```python
from build123d import *

# Parameters (mm, degrees)
SKETCH3_R           = 19.05
SKETCH3_R_2         = 2.159
BOSS_EXTRUDE1_DEPTH = 1.27


with BuildPart() as part:
    # Sketch2 → Revolve1 (revolve)
    with BuildSketch(Plane.XY, mode=Mode.PRIVATE) as revolve1_sk:
        Polygon((3.302, 35.814), (4.953, 35.814), (4.953, 28.702), (19.05, 28.702), (19.05, 18.669), (19.05, 17.399), (19.05, 7.366), (3.302, 7.366), align=None)
    revolve(revolve1_sk.sketch.rotate(Axis((0, 35.814, 0), (0, -1, 0)), 180), axis=Axis((0, 35.814, 0), (0, -1, 0)))

    # Sketch3 → Boss-Extrude1 (add)
    with BuildSketch(Plane(origin=(0, 17.399, 0), x_dir=(1, 0, 0), z_dir=(0, 1, 0))):
        with BuildLine():
            Line((-17.526, 22.225), (17.526, 22.225))
            ThreePointArc((17.526, 22.225), (20.848694765, 20.848694765), (22.225, 17.526))
            Line((22.225, 17.526), (22.225, -17.526))
            ThreePointArc((22.225, -17.526), (20.848694765, -20.848694765), (17.526, -22.225))
            Line((17.526, -22.225), (-17.526, -22.225))
            ThreePointArc((-17.526, -22.225), (-20.848694765, -20.848694765), (-22.225, -17.526))
            Line((-22.225, -17.526), (-22.225, 17.526))
            ThreePointArc((-22.225, 17.526), (-20.848694765, 20.848694765), (-17.526, 22.225))
        make_face()
        with Locations(Location((0, 0, 0), (0, 0, 180))):
            Circle(SKETCH3_R, mode=Mode.SUBTRACT)
        with Locations(Location((-17.526, -17.526, 0), (0, 0, 270))):
            Circle(SKETCH3_R_2, mode=Mode.SUBTRACT)
        with Locations(Location((17.526, -17.526, 0), (0, 0, 270))):
            Circle(SKETCH3_R_2, mode=Mode.SUBTRACT)
        with Locations(Location((-17.526, 17.526, 0), (0, 0, 270))):
            Circle(SKETCH3_R_2, mode=Mode.SUBTRACT)
        with Locations(Location((17.526, 17.526, 0), (0, 0, 270))):
            Circle(SKETCH3_R_2, mode=Mode.SUBTRACT)
    extrude(amount=BOSS_EXTRUDE1_DEPTH)


solid = part.part
```
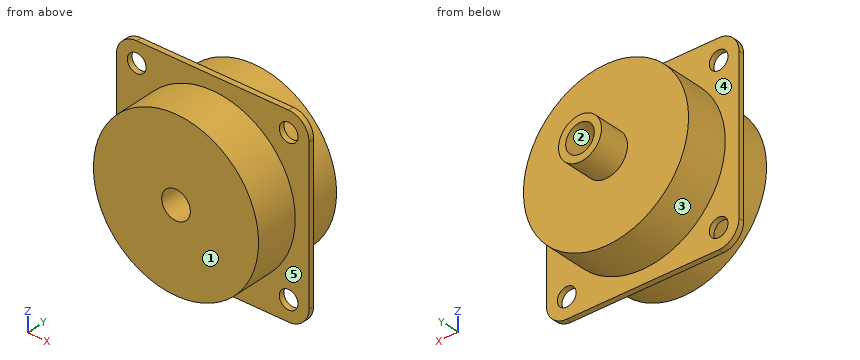
For this review, take the finished solid that the model builds, in its own axes (mm). Face numbers are marked on the shaded views. A direction names the side the tool comes from. Give positions to 0.01 mm unless a question says otherwise; leave off trailing zeros. Loops run counter-clockwise (first coordinate to the right, second up) from the corner with the lowest first, then second, coordinate; pieces in that order, holes last. Notation, with made-up numbers: M -26,-39 L 26,-39 A23 ccw 26,-22 Z; hole C 60.5,26 d8. An arc over 180 degrees is marked long. One line per item, written item: value. Start each with the question number.
Q1. Machinability: for the marked faces 4 and 5, which of the approach directions +Z, -Z, +X, -X, +Y, -Y give a long, thin tool a straight path to every point of the face, cutting with its end or side? Answer none if there is none.
Q2. Add section D-D (z = -9). Give the boundary of the cut face in (x, y) (3 decimals).
Q3. Add section B-B (z = 0). Give the boundary of the cut face in (x, y) (3 decimals), and give its area (3 significant figures).
Q4. Draft analysis for pull direction Z (two halves, no side actions). For the marked faces 1, 2 and 3, state which applies: released by +Z, released by -Z, zero draft, split by the parting line, or undercut.
Q5. Add section A-A (x = 0). Give the boundary of the cut face in (y, z) (3 decimals), and give its area (3 significant figures).
Q6. Clearance check with flat-ended pins moving along their axes: pin 1 Ø4 at (y, z) = (29, -6) entering from +X; pin 2 Ø5.5 at (x, z) = (17.526, 17.526) entering from -Y; pin 3 Ø8 at (y, z) = (30.5, -4.5) entering from -X; pin 4 Ø3.5 at (x, z) = (-17.526, 17.526) entering from +Y. State where each tip first meets the part, or that it passes through.
Q7. Add section C-C (y = 23). Give the boundary of the cut face in (x, z).
Q8. For L1, parallel to Y at x = -15, z = -20; L2, parallel to Y at x = 5, z = 8.5; L3, parallel to Z at x = 18, y = 18, list the stretches that pass through material, from the lowest coordinate up.
Reply:
1. face 4: +Y
1. face 5: -Y
2. outline: M -22.225,17.399 L -16.79,17.399 L -16.79,7.366 L 16.79,7.366 L 16.79,17.399 L 22.225,17.399 L 22.225,18.669 L 16.79,18.669 L 16.79,28.702 L -16.79,28.702 L -16.79,18.669 L -22.225,18.669 Z
3. outline: M -22.225,17.399 L -19.05,17.399 L -19.05,7.366 L -3.302,7.366 L -3.302,35.814 L -4.953,35.814 L -4.953,28.702 L -19.05,28.702 L -19.05,18.669 L -22.225,18.669 Z; M 3.302,7.366 L 19.05,7.366 L 19.05,17.399 L 22.225,17.399 L 22.225,18.669 L 19.05,18.669 L 19.05,28.702 L 4.953,28.702 L 4.953,35.814 L 3.302,35.814 Z
3. area: 704 mm²
4. face 1: zero draft
4. face 2: undercut
4. face 3: split by the parting line
5. outline: M 7.366,-19.05 L 17.399,-19.05 L 17.399,-22.225 L 18.669,-22.225 L 18.669,-19.05 L 28.702,-19.05 L 28.702,-4.953 L 35.814,-4.953 L 35.814,-3.302 L 7.366,-3.302 Z; M 7.366,3.302 L 35.814,3.302 L 35.814,4.953 L 28.702,4.953 L 28.702,19.05 L 18.669,19.05 L 18.669,22.225 L 17.399,22.225 L 17.399,19.05 L 7.366,19.05 Z
5. area: 704 mm²
6. pin 1: x = 18.62
6. pin 2: y = 17.4
6. pin 3: x = -19.03
6. pin 4: through
7. outline: C 0,0 d38.1; hole C 0,0 d6.6
8. L1: 17.4 to 18.67
8. L2: 7.37 to 28.7
8. L3: -22.2 to -19.63, -15.42 to 15.42, 19.63 to 22.2
